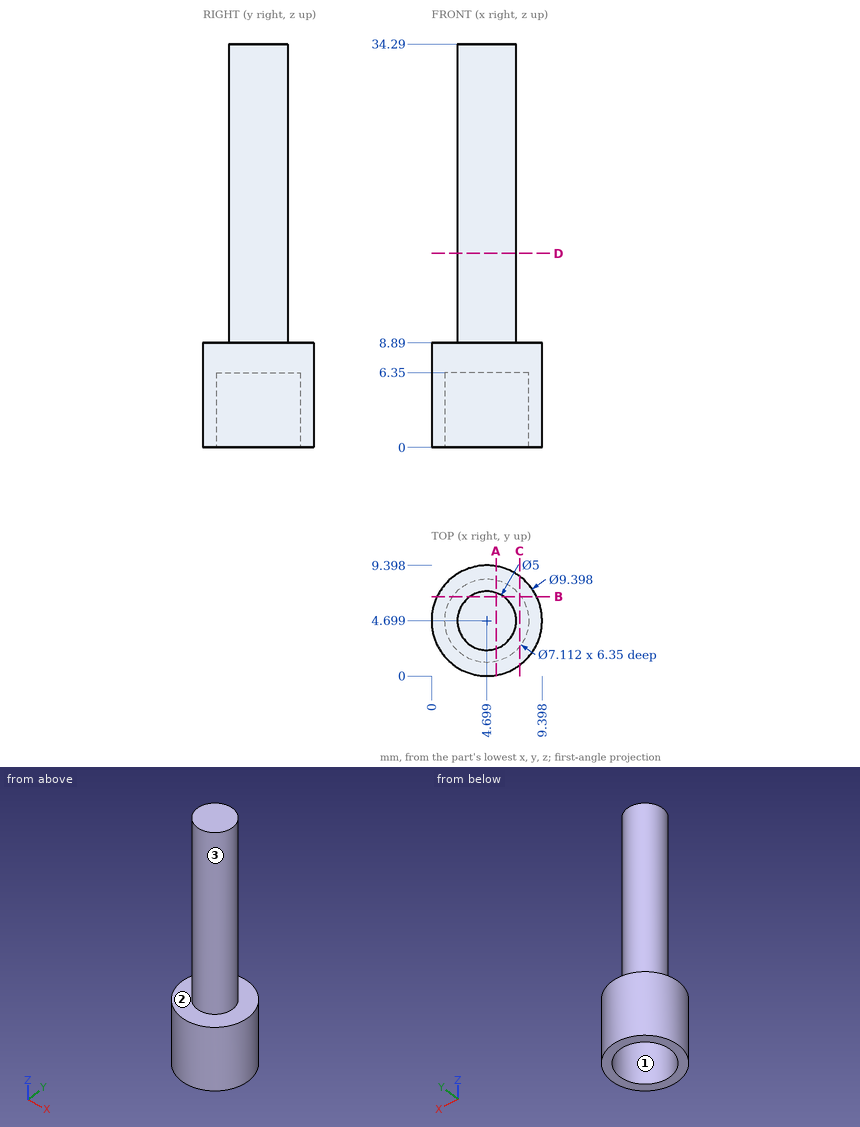
Geometry check sheet. Reference: drawing and pictorial views, mm from the part's lowest x, y, z. Give positions to 0.01 mm unless a question says otherwise; leave off trailing zeros. Loops run counter-clockwise (first coordinate to the right, second up) from the corner with the lowest first, then second, coordinate; pieces in that order, holes last. Notation, with made-up numbers: M -26,-16.75 L -4,-16.75 A7 cw -4,-7.75 Z; hole C -11,15.5 d1. An arc over 180 degrees is marked long. Use a Markdown table: item, result. Add a question column.
Q1. Sectioned sample at B-B, the plane y = 6.75. Record the cut outline in (x, z).
Q2. Mould release check, pull along X, two halves, no side actions. Record for the marked faces 1, 2 and 3: pulls with the +X half, pulls with the -X half, needs draft (parallel to the pull), parting line crosses it, or undercut.
Q3. Sectioned sample at A-A, the plane x = 5.5. Record the cut outline in (y, z), then the cut area to 3 significant figures.
Q4. Sectioned sample at C-C, the plane x = 7.5. Record the cut outline in (y, z).
Q5. Go/stop test with flat-tipped pins: pin 1 (2 mm diameter, centred on x = 2.5, z = 7.5, fed in from -Y); pin 2 (2 mm diameter, centred on x = 7.5, z = 11, fed in from -Y); pin 3 (1.5 mm diameter, centred on x = 3, y = 6.5, fed in from -Z). Record where each tip stops, or that it passes through.
Q6. Scan lines: line 1 along Z through (x, y) = (2.5, 3.25); line 2 along Z through (x, y) = (4.25, 3.5); line 3 along Y through (x, z) = (7.25, 6). Record each from-to range of solid material in increasing order. Write a range as [from, to].
Q7. Sectioned sample at D-D, the plane z = 16.5. Record the cut outline in (x, y).
Verdict:
| question | item | result |
|---|---|---|
| 1 | outline | M 0.47,0 L 1.79,0 L 1.79,6.35 L 7.6,6.35 L 7.6,0 L 8.93,0 L 8.93,8.89 L 6.13,8.89 L 6.13,34.29 L 3.27,34.29 L 3.27,8.89 L 0.47,8.89 Z |
| 2 | face 1 | undercut |
| 2 | face 2 | needs draft |
| 2 | face 3 | parting line crosses it |
| 3 | outline | M 0.07,0 L 1.23,0 L 1.23,6.35 L 8.16,6.35 L 8.16,0 L 9.33,0 L 9.33,8.89 L 7.07,8.89 L 7.07,34.29 L 2.33,34.29 L 2.33,8.89 L 0.07,8.89 Z |
| 3 | area | 159 mm^2 |
| 4 | outline | M 0.93,0 L 2.51,0 L 2.51,6.35 L 6.89,6.35 L 6.89,0 L 8.47,0 L 8.47,8.89 L 0.93,8.89 Z |
| 5 | pin 1 | y = 0.16 |
| 5 | pin 2 | y = 2.97 |
| 5 | pin 3 | z = 6.35 |
| 6 | line 1 | [6.35, 8.89] |
| 6 | line 2 | [6.35, 34.29] |
| 6 | line 3 | [0.75, 2.22], [7.18, 8.65] |
| 7 | outline | C 4.7,4.7 d5 |
